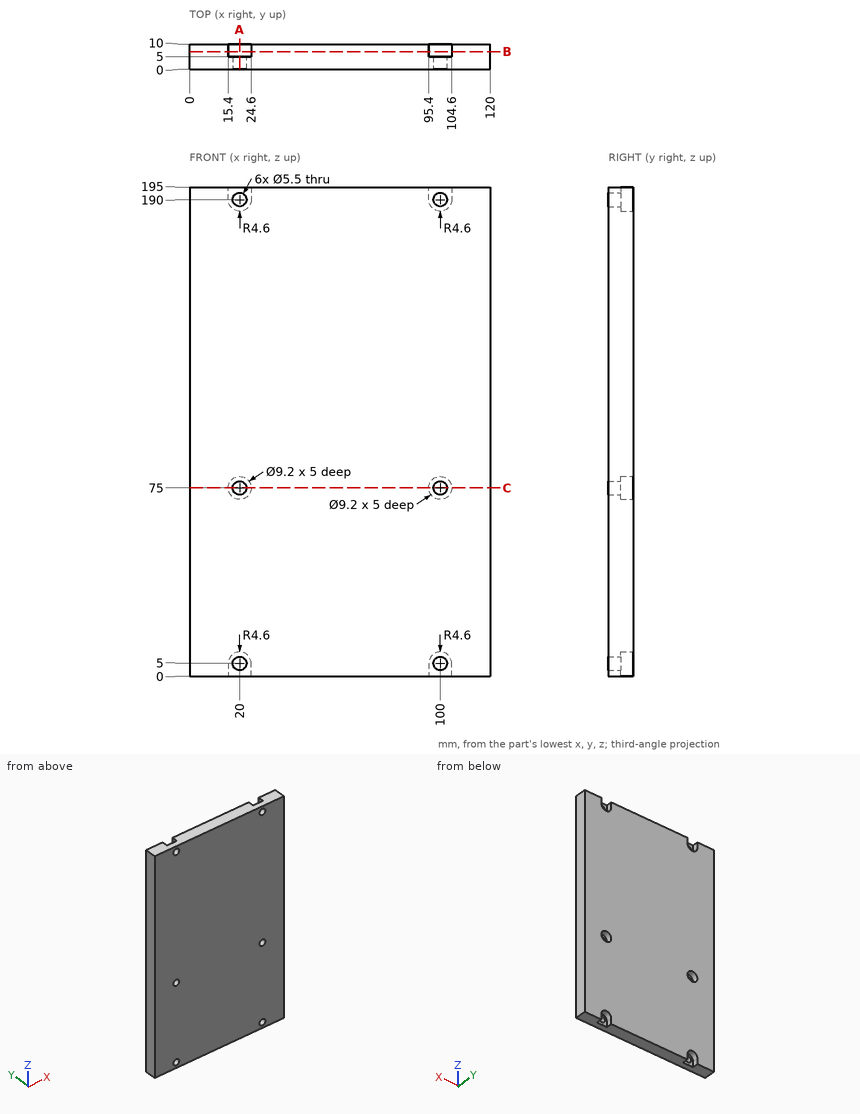
Verification items for this drawing (mm, ordinates from the low corner). Give positions to 0.01 mm unless a question says otherwise; leave off trailing zeros. Write each loop counter-clockwise with the first axis right and the second up, starting at its lowest first coordinate (ties: lowest second). Pieces come first, ordered by that corner, then holes.
1) Cross-section at C-C (z = 75). Record the boundary of the cut face in (x, y), plus the area to 3 significant figures.
Values follow:
outline: (0, 0) - (17.25, 0) - (17.25, 5) - (15.4, 5) - (15.4, 10) - (0, 10) - close; (22.75, 0) - (97.25, 0) - (97.25, 5) - (95.4, 5) - (95.4, 10) - (24.6, 10) - (24.6, 5) - (22.75, 5) - close; (102.75, 0) - (120, 0) - (120, 10) - (104.6, 10) - (104.6, 5) - (102.75, 5) - close
area: 1,050 mm2
2) Cross-section at A-A (x = 20). Record the boundary of the cut face in (y, z).
Values follow:
outline: (0, 0) - (5, 0) - (5, 2.25) - (0, 2.25) - close; (0, 7.75) - (5, 7.75) - (5, 9.6) - (10, 9.6) - (10, 70.4) - (5, 70.4) - (5, 72.25) - (0, 72.25) - close; (0, 77.75) - (5, 77.75) - (5, 79.6) - (10, 79.6) - (10, 185.4) - (5, 185.4) - (5, 187.25) - (0, 187.25) - close; (0, 192.75) - (5, 192.75) - (5, 195) - (0, 195) - close
3) Go/stop test with flat-tipped pins: pin 1 Ø1.5 at (y, z) = (6.5, 3.5) entering from -X; pin 2 Ø5 at (x, z) = (20, 75) entering from -Y; pin 3 Ø4.5 at (x, z) = (21.5, 6) entering from +Y. Record where each tip stops, or that it passes through.
Values follow:
pin 1: stops at x = 0
pin 2: passes through
pin 3: stops at y = 5
4) Cross-section at B-B (y = 7). Record the boundary of the cut face in (x, z), plus the area to 3 significant figures.
Values follow:
outline: (0, 0) - (15.4, 0) - (15.4, 5) arc R4.6 cw to (24.6, 5) - (24.6, 0) - (95.4, 0) - (95.4, 5) arc R4.6 cw to (104.6, 5) - (104.6, 0) - (120, 0) - (120, 195) - (104.6, 195) - (104.6, 190) arc R4.6 cw to (95.4, 190) - (95.4, 195) - (24.6, 195) - (24.6, 190) arc R4.6 cw to (15.4, 190) - (15.4, 195) - (0, 195) - close; hole circle Ø9.2 at (20, 75); hole circle Ø9.2 at (100, 75)
area: 23,000 mm2
5) Thickness scan on line 1 (Z direction, x = 20, y = 3.95); line 2 (X direction, y = 2.25, z = 190); line 3 (X direction, y = 3.25, z = 74). Record the ranges inside material, lowest first.
Values follow:
line 1: z = 0 to 2.25, 7.75 to 72.25, 77.75 to 187.25, 192.75 to 195
line 2: x = 0 to 17.25, 22.75 to 97.25, 102.75 to 120
line 3: x = 0 to 17.44, 22.56 to 97.44, 102.56 to 120
